Verification items for the finished model (mm, model axes). A direction names the side the tool comes from. Round coordinates to 2 decimals unless told otherwise and drop trailing zeros. Loops run counter-clockwise (first coordinate to the right, second up) from the corner with the lowest first, then second, coordinate; pieces in that order, holes last. Notation, with made-up numbers: (40, 28) -> (76, 28) arc R24 ccw to (76, 61) -> close; hole circle Ø10 at (-34.5, 27.5). An arc over 180 degrees is marked (long way). Write item = value, one per line. Start each with the question number.
```python
from build123d import *

# Parameters (mm, degrees)
SKETCH_1_R          = 16
EXTRUDE_1_DEPTH     = 11
CHAMFER_1_SIZE      = 1
SKETCH_2_R          = 12
CUT_EXTRUDE_1_DEPTH = 8


with BuildPart() as part:
    # 草图1 → 拉伸1 (new body)
    with BuildSketch(Plane.XY):
        Circle(SKETCH_1_R)
    extrude(amount=EXTRUDE_1_DEPTH)

    # 倒角1
    chamfer_1_edges = [part.edges().sort_by_distance(p)[0] for p in [
        (-16, 0, 0),
        (-16, 0, 11),
    ]]
    chamfer(chamfer_1_edges, length=CHAMFER_1_SIZE)

    # 草图2 → 切除-拉伸1 (cut)
    with BuildSketch(Plane.XY.offset(11)):
        Circle(SKETCH_2_R)
    extrude(amount=-CUT_EXTRUDE_1_DEPTH, mode=Mode.SUBTRACT)


solid = part.part
```
(1) Scan lines: line 1 (Y direction, x = 0, z = 4.75); line 2 (Z direction, x = -6.5, y = -7.5); line 3 (Y direction, x = -3, z = 5.25). Record each from-to range of solid material in increasing order. Write a range as [from, to].
(2) Draft check along Y on faces 3 (the flat face through (0, 0, 3)), 4 (the cylindrical face through (-3.47, -15.62, 5.44)), 5 (the flat face through (-7, 10, 11)). Enter one of: +Y half, -Y half, draft (parallel to the pull), parting line (faces both ways), or undercut.
(3) Section check A-A on x = 0. Enter the section's corners in (y, z), then the cut area to 3 significant figures.
(4) Section check C-C on z = 5.5. Enter the section's corners in (x, y).
(5) Depth check by flat-ended pin: pin 1 Ø1.5 at (x, z) = (-7, 1.5) entering from -Y; pin 2 Ø7 at (x, y) = (-0.5, 2) entering from +Z; pin 3 Ø3 at (y, z) = (11, 1.5) entering from +X. Enter the tip coordinate at first touch or a pass-through.
(6) Access from +Z, -Z, +X, -X, +Y, -Y to the whole of each face (thin tool, end or side, straight path). Record for faces 1 (the flat face through (0, 0, 0)), 2 (the cylindrical face through (-11.99, 0.53, 7.06)).
(7) Section check D-D on z = 2.5. Enter the section's corners in (x, y), then the cut area to 3 significant figures.
Computed values:
q1.line_1 = [-16, -12], [12, 16]
q1.line_2 = [0, 3]
q1.line_3 = [-15.72, -11.62], [11.62, 15.72]
q2.face_3 = undercut
q2.face_4 = parting line
q2.face_5 = draft
q3.outline = (-16, 1) -> (-15, 0) -> (15, 0) -> (16, 1) -> (16, 10) -> (15, 11) -> (12, 11) -> (12, 3) -> (-12, 3) -> (-12, 11) -> (-15, 11) -> (-16, 10) -> close
q3.area = 158 mm²
q4.outline = circle Ø32 at (0, 0); hole circle Ø24 at (0, 0)
q5.pin_1 = -14.73
q5.pin_2 = 3
q5.pin_3 = 12.87
q6.face_1 = -Z, +X, -X, +Y, -Y
q6.face_2 = +Z
q7.outline = circle Ø32 at (0, 0)
q7.area = 804 mm²
